Read the model definition and answer for the solid it produces. Units are mm, in the model's axes. Round coordinates to 2 decimals unless told otherwise and drop trailing zeros. Write each loop counter-clockwise with the first axis right and the second up, starting at its lowest first coordinate (ties: lowest second). Pieces come first, ordered by that corner, then holes. Notation, with made-up numbers: (24, -18) - (40, -18) arc R16 cw to (40, 1) - close; hole circle Ø9 at (12, 74.25). An arc over 180 degrees is marked (long way). One line per item, written item: value. Start each with the question number.
(1) A cutting plane is placed at B-B, the plane x = 20.5. Determine the outline of the cut face in (y, z), plus the area to 3 significant figures.
(2) A flat-ended cylindrical pin translates along its axis: pin 1 Ø2 at (x, z) = (-24, 0.5) entering from -Y. Find the tip coordinate at first contact, or state that the pin passes through.
(3) Find the intervals of material crossed by L1, parallel to Z at x = -1, y = 0.7; L2, parallel to Y at x = -7.5, z = 1.4; L3, parallel to Z at x = 19, y = 1.3, in increasing order.
(4) A cutting plane is placed at A-A, the plane x = 0.5. Determine the outline of the cut face in (y, z).
from build123d import *

# Parameters (mm, degrees)
CHAMFER1_SIZE = 0.2


with BuildPart() as part:
    # Sketch1 → Revolve1 (revolve)
    with BuildSketch(Plane.XY, mode=Mode.PRIVATE) as revolve1_sk:
        with BuildLine():
            Line((-30, 0), (30, 0))
            Line((30, 0), (30, 1))
            Line((30, 1), (21, 1))
            ThreePointArc((21, 1), (20.146606905, 1.145068441), (19.317048796, 1.392369816))
            ThreePointArc((19.317048796, 1.392369816), (17.627383867, 1.846920792), (15.884354631, 2))
            Line((15.884354631, 2), (-15.884354631, 2))
            ThreePointArc((-15.884354631, 2), (-17.60385956, 1.851055923), (-19.272142474, 1.40866056))
            ThreePointArc((-19.272142474, 1.40866056), (-20.124476001, 1.155304466), (-21, 1))
            Line((-21, 1), (-30, 1))
            Line((-30, 1), (-30, 0))
        make_face()
    revolve(revolve1_sk.sketch.rotate(Axis((-30, 0, 0), (1, 0, 0)), 180), axis=Axis((-30, 0, 0), (1, 0, 0)))

    # Chamfer1
    chamfer1_edges = [part.edges().sort_by_distance(p)[0] for p in [
        (30, 1, 0),
        (-30, 1, 0),
    ]]
    chamfer(chamfer1_edges, length=CHAMFER1_SIZE)


solid = part.part
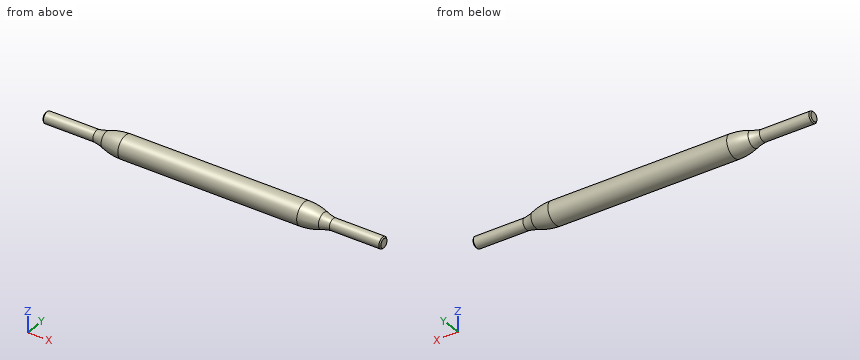
Here are the results:
1. outline: circle Ø2.14 at (0, 0)
1. area: 3.61 mm²
2. pin 1: y = -1
3. L1: -1.87 to 1.87
3. L2: -1.43 to 1.43
3. L3: -0.75 to 0.75
4. outline: circle Ø4 at (0, 0)
